```python
from build123d import *

# Parameters (mm, degrees)
F3_R      = 3.75
F4_DEPTH  = 7.5
F6_R      = 2.25
F7_DEPTH  = 17.001
F9_R      = 3.5
F10_DEPTH = 25


# Not quite as in the source:
# - a fillet or chamfer that OpenCascade refuses, or shapes differently, is made with other operations: its cross-section is extruded or revolved along the edge and cut away or added


with BuildPart() as f1:
    # F0 (on Front) → F1 (revolve)
    with BuildSketch(Plane.XZ):
        with BuildLine():
            Line((0, 0), (17, 0))
            ThreePointArc((17, 0), (12.0208152802, 12.0208152802), (0, 17))
            Line((0, 17), (0, 0))
        make_face()
    revolve(axis=Axis((0, 0, 8.5), (0, 0, 1)))

    # F3 (on offset) → F4 (cut, symmetric)
    with BuildSketch(Plane.XZ.offset(15)):
        with Locations((-8, 6)):
            Circle(F3_R)
        with Locations((8, 6)):
            Circle(F3_R)
    extrude(amount=F4_DEPTH, both=True, mode=Mode.SUBTRACT)

    # F5: chamfer of 1 on 1 edges, made by hand

    # F5_s1 → F5_t2 (revolve, cut)
    with BuildSketch(Plane.XZ):
        with BuildLine():
            Line((15.9687194227, 0), (16.9667643866, 1.0625))
            ThreePointArc((16.9667643866, 1.0625), (16.9912411836, 0.54564003), (17, 0))
            Line((17, 0), (15.9687194227, 0))
        make_face()
    revolve(axis=Axis((0, 0, 0), (0, 0, 1)), mode=Mode.SUBTRACT)

    # F6 (on Top) → F7 (cut, through all)
    with BuildSketch(Plane.XY):
        Circle(F6_R)
    extrude(amount=F7_DEPTH, mode=Mode.SUBTRACT)

    # F9 (on offset) → F10 (cut)
    with BuildSketch(Plane.XY.offset(30)):
        Circle(F9_R)
    extrude(amount=-F10_DEPTH, mode=Mode.SUBTRACT)


solid = f1.part
```
For this review, take the finished solid that the model builds, in its own axes (mm). A direction names the side the tool comes from. Round coordinates to 2 decimals unless told otherwise and drop trailing zeros. Write each loop counter-clockwise with the first axis right and the second up, starting at its lowest first coordinate (ties: lowest second). Pieces come first, ordered by that corner, then holes. Notation, with made-up numbers: (68.5, 50) - (125.5, 50) arc R32 cw to (125.5, 77) - close; hole circle Ø9 at (39, 63.25). An arc over 180 degrees is marked (long way). Answer as a JSON object with one key per item and string values.
1. We need section A-A on y = 0. Give the boundary of the cut face in (x, z).
Response values:
{"outline": "(-16.97, 1.06) - (-15.97, 0) - (-2.25, 0) - (-2.25, 5) - (-3.5, 5) - (-3.5, 16.64) arc R17 ccw to start; (2.25, 0) - (15.97, 0) - (16.97, 1.06) arc R17 ccw to (3.5, 16.64) - (3.5, 5) - (2.25, 5) - close"}
2. Draft analysis for pull direction Y (two halves, no side actions). For faces 1 (the face through (0.7, -2.3, 5)), 2 (the face through (3.233, -1.341, 10.899)), 3 (the face through (0, -3, 0)), 4 (the face through (8, -7.5, 6)), state which applies: +Y half, -Y half, draft (parallel to the pull), parting line (faces both ways), or undercut.
Response values:
{"face 1": "undercut", "face 2": "undercut", "face 3": "draft", "face 4": "-Y half"}
3. Tool access review of faces 5 (the face through (-8, -7.5, 6)), 6 (the face through (-0.29, 2.23, 2.46)): name each direction out of +Z, -Z, +X, -X, +Y, -Y from which nothing blocks a thin tool from reaching the whole face with its end or side.
Response values:
{"face 5": "-Y", "face 6": "+Z, -Z"}
4. We need section D-D on z = 11.5. Give the boundary of the cut face in (x, y).
Response values:
{"outline": "circle Ø25.04 at (0, 0); hole circle Ø7 at (0, 0)"}
5. To check wall thickness, follow line 1 along X through (y, z) = (0, 12); line 2 along Y through (x, z) = (2, 5.5); line 3 along X through (y, z) = (0, 9). State the ranges of each line that lie inside material, in increasing order.
Response values:
{"line 1": "x = -12.04 to -3.5, 3.5 to 12.04", "line 2": "y = -15.96 to -2.87, 2.87 to 15.96", "line 3": "x = -14.42 to -3.5, 3.5 to 14.42"}
6. We need section C-C on z = 2.75. Give the boundary of the cut face in (x, y), then the cut area to 3 significant figures.
Response values:
{"outline": "(-9.87, -13.56) - (-9.87, -7.5) - (-6.13, -7.5) - (-6.13, -15.62) arc R16.78 ccw to (6.13, -15.62) - (6.13, -7.5) - (9.87, -7.5) - (9.87, -13.56) arc R16.78 ccw (long way) to start; hole circle Ø4.5 at (0, 0)", "area": "814 mm2"}
7. For pin 1 Ø9 at (x, y) = (0, 0) entering from -Z; pin 2 Ø8 at (x, z) = (-9, 7) entering from -Y; pin 3 Ø4 at (y, z) = (-3, 15) entering from -X; pin 4 Ø4 at (x, z) = (3, 10.5) entering from -Y, all flat-tipped, find the tip position at first contact; note any pin that passes through.
Response values:
{"pin 1": "stops at z = 0", "pin 2": "stops at y = -13.61", "pin 3": "stops at x = -10.59", "pin 4": "stops at y = -14.47"}
